Build history of the part. All positions in model axes, mm. A direction names the side the tool comes from. Round coordinates to 2 decimals unless told otherwise and drop trailing zeros. Write each loop counter-clockwise with the first axis right and the second up, starting at its lowest first coordinate (ties: lowest second). Pieces come first, ordered by that corner, then holes.
Item 1: Band-saw the part on D-D, the plane z = 6.75. Write the cut outline in (x, y).
Item 2: Band-saw the part on B-B, the plane y = 0. Write the cut outline in (x, z).
Item 3: 3-axis set-ups, long thin cutter, end or side, ignore diameter. For faces 1 (the flat face through (1, 6.5, 0)), 2 (the flat face through (1, 6, 2)), 3 (the cylindrical face through (1, -5, 0)), 4 (the flat face through (1, 6, -2)), 5 (the cylindrical face through (7.36, -1.08, 4.88)): which of +Z, -Z, +X, -X, +Y, -Y reach the whole face in a straight line?
Item 4: Band-saw the part on A-A, the plane z = 0. Write the cut outline in (x, y), then the cut area to 3 significant figures.
Item 5: Drop flat-ended pins along their axis: pin 1 Ø1 at (y, z) = (-2.5, 1) entering from -X; pin 2 Ø0.6 at (x, y) = (1, 5) entering from +Z; pin 3 Ø2 at (x, z) = (0.5, 0) entering from +Y; pin 4 Ø4 at (x, y) = (7.5, 3) entering from +Z. Give the stop position or say it passes through.
Item 6: Band-saw the part on C-C, the plane x = 2.75. Write the cut outline in (y, z).
Item 7: Wall check: probe 1 along X at (y, z) = (3.75, 4.25); probe 2 along Z at (x, y) = (6, 0); probe 3 along Z at (x, y) = (2.25, -1.25). Give the ranges that are in metal, low to high.
Autodesk Inventor part; units mm, degrees
ref_plane "YZ Plane" through (0, 0, 0) normal (1, 0, 0) x (0, 1, 0)
ref_plane "XZ Plane" through (0, 0, 0) normal (0, 1, 0) x (-1, 0, 0)
ref_plane "XY Plane" through (0, 0, 0) normal (0, 0, 1) x (1, 0, 0)
sketch "Sketch1" plane through (0, 0, 0) normal (1, 0, 0) x (0, 1, 0)
  circle A0 centre (0, 0) radius 5
  dimension "d0" = 10
extrude "Extrusion1" add sketch "Sketch1" along normal blind 10
sketch "Sketch2" plane through (0, 0, 0) normal (-1, 0, 0) x (0, 0, 1)
  circle A0 centre (0, 0) radius 5
  line L0 (-2, 6.5) -> (2, 6.5)
  line L1 (2, 6.5) -> (2, 0)
  line L2 (2, 0) -> (-2, 0)
  line L3 (-2, 0) -> (-2, 6.5)
  point P0 (0, -5)
  point P1 (-2, 4.5826)
  point P2 (2, 4.5826)
  dimension "d3" = 11.5
  dimension "d4" = 4
extrude "Extrusion2" add sketch "Sketch2" against normal blind 2 contours A0 L3 L0 L1
sketch "Sketch3" plane through (2, 0, 0) normal (1, 0, 0) x (0, 0, -1)
  circle A0 centre (0, 0) radius 7.5
  dimension "d7" = 15
extrude "Extrusion3" add sketch "Sketch3" along normal blind 2.8
properties part number "PIEZA_AYUDA" material "Steel, Mild, Welded"
Results:
1. outline: (2, -3.27) - (4.8, -3.27) - (4.8, 3.27) - (2, 3.27) - close
2. outline: (0, -5) - (2, -5) - (2, -7.5) - (4.8, -7.5) - (4.8, -5) - (10, -5) - (10, 5) - (4.8, 5) - (4.8, 7.5) - (2, 7.5) - (2, 5) - (0, 5) - close
3. face 1: +Z, -Z, -X, +Y
3. face 2: +Z, -X, +Y
3. face 3: -X
3. face 4: -Z, -X, +Y
3. face 5: +X
4. outline: (0, -5) - (2, -5) - (2, -7.5) - (4.8, -7.5) - (4.8, -5) - (10, -5) - (10, 5) - (4.8, 5) - (4.8, 7.5) - (2, 7.5) - (2, 6.5) - (0, 6.5) - close
4. area: 117 mm2
5. pin 1: stops at x = 0
5. pin 2: stops at z = 2
5. pin 3: stops at y = 6.5
5. pin 4: stops at z = 4.9
6. outline: circle Ø15 at (0, 0)
7. probe 1: x = 2 to 4.8
7. probe 2: z = -5 to 5
7. probe 3: z = -7.4 to 7.4
